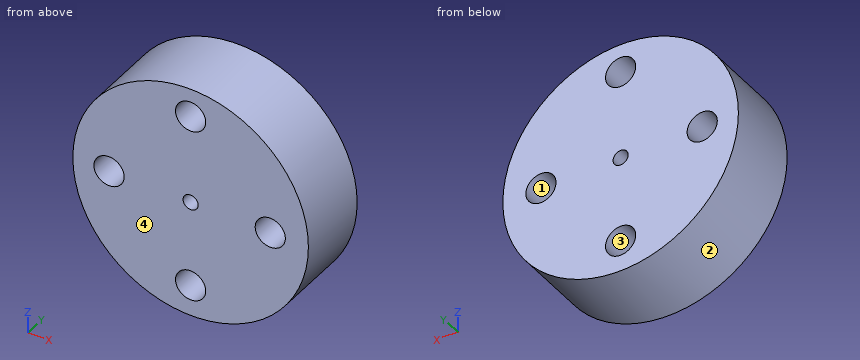
Autodesk Inventor part; units mm, degrees
ref_plane "YZ Plane" through (0, 0, 0) normal (1, 0, 0) x (0, 1, 0)
ref_plane "XZ Plane" through (0, 0, 0) normal (0, 1, 0) x (-1, 0, 0)
ref_plane "XY Plane" through (0, 0, 0) normal (0, 0, 1) x (1, 0, 0)
sketch "Sketch1" plane through (0, 0, 0) normal (0, 1, 0) x (-1, 0, 0)
  circle A0 centre (0, 0) radius 39
  circle A1 centre (0, 0) radius 2.5
  circle A2 centre (27.0171, 0) radius 5
  circle A3 centre (0, -28.6186) radius 5
  circle A4 centre (-26.381, 0) radius 5
  circle A5 centre (0, 29.5447) radius 5
  dimension "d0" = 78
  dimension "d1" = 5
  dimension "d2" = 10
  dimension "d3" = 10
  dimension "d4" = 10
  dimension "d5" = 10
extrude "Extrusion1" add sketch "Sketch1" along normal blind 25
properties part number "roller1 grp17"
Geometry check sheet. Reference: the model listing, model coordinates, mm. Face numbers are marked on the shaded views. Give positions to 0.01 mm unless a question says otherwise; leave off trailing zeros. Loops run counter-clockwise (first coordinate to the right, second up) from the corner with the lowest first, then second, coordinate; pieces in that order, holes last. Notation, with made-up numbers: M -25.75,79.5 L -11.75,79.5 A37 ccw -11.75,115.5 Z; hole C 6,55 d8. An arc over 180 degrees is marked long. Answer as a JSON object with one key per item and string values. Group by question number.
Item 1: Sectioned sample at C-C on z = -26. Record the boundary of the cut face in (x, y).
Item 2: Gauge pin test, flat ends, axial feed: pin 1 (6 mm diameter, centred on x = -27.02, z = 0, fed in from +Y); pin 2 (2 mm diameter, centred on x = 21, y = 8.5, fed in from +Z); pin 3 (1.5 mm diameter, centred on y = 3.5, z = -28, fed in from +X); pin 4 (3 mm diameter, centred on y = 7, z = -27.5, fed in from +X). Record the tip position at first contact, or that the pin passes through.
Item 3: Sectioned sample at D-D on y = 3. Record the boundary of the cut face in (x, z), plus the area to 3 significant figures.
Item 4: Sectioned sample at A-A on z = 0. Record the boundary of the cut face in (x, y).
Item 5: Material ranges on L1, parallel to Z at x = 0, y = 10.25; L2, parallel to Z at x = 3, y = 16; L3, parallel to Z at x = -2, y = 12.5, recorded low to high.
Item 6: Sectioned sample at B-B on x = 0. Record the boundary of the cut face in (y, z), plus the area to 4 significant figures.
Item 7: Mould release check, pull along Z, two halves, no side actions. Record for the marked faces 1, 2, 3 and 4: pulls with the +Z half, pulls with the -Z half, needs draft (parallel to the pull), parting line crosses it, or undercut.
Findings below:
{
 "1": {"outline": "M -29.07,0 L -4.26,0 L -4.26,25 L -29.07,25 Z; M 4.26,0 L 29.07,0 L 29.07,25 L 4.26,25 Z"},
 "2": {"pin 1": "through", "pin 2": "z = 33.48", "pin 3": "x = 27.9", "pin 4": "x = 29.07"},
 "3": {"outline": "C 0,0 d78; hole C -27.02,0 d10; hole C 0,-28.62 d10; hole C 0,29.54 d10; hole C 0,0 d5; hole C 26.38,0 d10", "area": "4,440 mm2"},
 "4": {"outline": "M -39,0 L -32.02,0 L -32.02,25 L -39,25 Z; M -22.02,0 L -2.5,0 L -2.5,25 L -22.02,25 Z; M 2.5,0 L 21.38,0 L 21.38,25 L 2.5,25 Z; M 31.38,0 L 39,0 L 39,25 L 31.38,25 Z"},
 "5": {"L1": "-39 to -33.62, -23.62 to -2.5, 2.5 to 24.54, 34.54 to 39", "L2": "-38.88 to -32.62, -24.62 to 25.54, 33.54 to 38.88", "L3": "-38.95 to -33.2, -24.04 to -1.5, 1.5 to 24.96, 34.13 to 38.95"},
 "6": {"outline": "M 0,-39 L 25,-39 L 25,-33.62 L 0,-33.62 Z; M 0,-23.62 L 25,-23.62 L 25,-2.5 L 0,-2.5 Z; M 0,2.5 L 25,2.5 L 25,24.54 L 0,24.54 Z; M 0,34.54 L 25,34.54 L 25,39 L 0,39 Z", "area": "1,325 mm2"},
 "7": {"face 1": "undercut", "face 2": "parting line crosses it", "face 3": "undercut", "face 4": "needs draft"}
}
